Drawing for the job (mm, zero at the part's lowest x, y, z). Give positions to 0.01 mm unless a question says otherwise; leave off trailing zeros. Order: outer loops, then holes, each group sorted by start corner. A loop starts at its lowest first (then second) coordinate and runs counter-clockwise, first axis right, second up. Notation, with made-up numbers: (88, 60.5) -> (131, 60.5) arc R31 cw to (131, 84.5) -> close; hole circle Ø2 at (75, 65). An arc over 180 degrees is marked (long way). Use one line per item in the form item = value. Start each with the question number.
1) Cut at B-B, the plane y = 8. Give the cut face in (x, z).
2) Mould opens along X. For the marked faces 1, 2, 3 and 4 say: pulls with the +X half, pulls with the -X half, needs draft (parallel to the pull), parting line crosses it, or undercut.
3) Cut at D-D, the plane x = 7. Give the cut face in (y, z), and give its area (3 significant figures).
4) Cut at C-C, the plane z = 7.25. State how many separate pieces and enclosed holes the cut face has, and give its area (3 significant figures).
5) Probe line 1 (Y direction, x = 16, z = 3.5); line 2 (Y direction, x = 54, z = 0.75); line 3 (X direction, y = 7, z = 5). List the from-to ranges inside material, lowest first.
6) Drop flat-ended pins along their axis: P1, Ø2, axis at y = 12, z = 4, coming from the -X side; P2, Ø4.5, axis at x = 6, y = 8, coming from the +Z side. Give the stop position or say it passes through.
7) Cut at A-A, the plane x = 44. Give the cut face in (y, z).
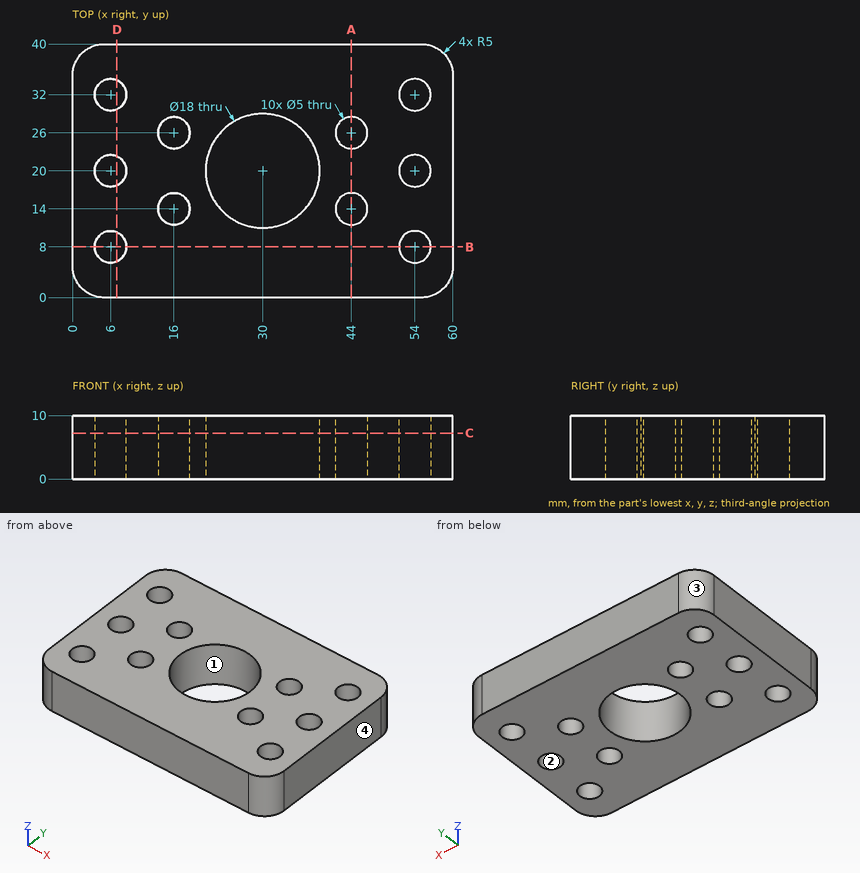
Result:
q1.outline = (0, 0) -> (3.5, 0) -> (3.5, 10) -> (0, 10) -> close; (8.5, 0) -> (51.5, 0) -> (51.5, 10) -> (8.5, 10) -> close; (56.5, 0) -> (60, 0) -> (60, 10) -> (56.5, 10) -> close
q2.face_1 = undercut
q2.face_2 = undercut
q2.face_3 = pulls with the -X half
q2.face_4 = pulls with the +X half
q3.outline = (0, 0) -> (5.71, 0) -> (5.71, 10) -> (0, 10) -> close; (10.29, 0) -> (17.71, 0) -> (17.71, 10) -> (10.29, 10) -> close; (22.29, 0) -> (29.71, 0) -> (29.71, 10) -> (22.29, 10) -> close; (34.29, 0) -> (40, 0) -> (40, 10) -> (34.29, 10) -> close
q3.area = 263 mm²
q4.separate_pieces = 1
q4.enclosed_holes = 11
q4.area = 1,930 mm²
q5.line_1 = 0 to 11.5, 16.5 to 23.5, 28.5 to 40
q5.line_2 = 0 to 5.5, 10.5 to 17.5, 22.5 to 29.5, 34.5 to 40
q5.line_3 = 0 to 3.71, 8.29 to 51.71, 56.29 to 60
q6.P1 = 0
q6.P2 = through
q7.outline = (0, 0) -> (11.5, 0) -> (11.5, 10) -> (0, 10) -> close; (16.5, 0) -> (23.5, 0) -> (23.5, 10) -> (16.5, 10) -> close; (28.5, 0) -> (40, 0) -> (40, 10) -> (28.5, 10) -> close
